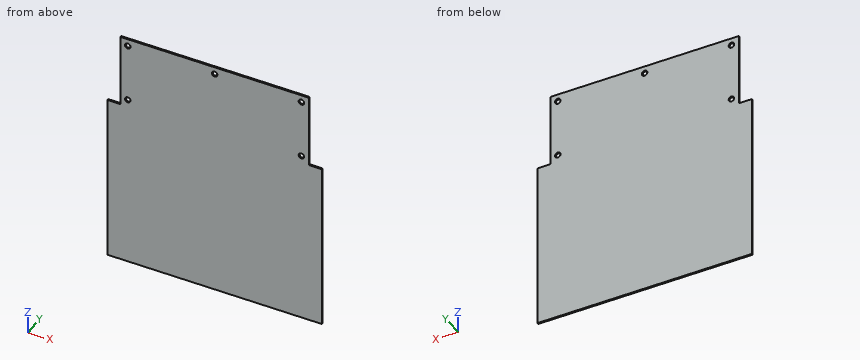
from build123d import *

# Parameters (mm, degrees)
F0_R     = 3.25
F1_DEPTH = 2
F2_SIZE  = 0.5


with BuildPart() as f1:
    # F0 (on Front) → F1 (new body)
    with BuildSketch(Plane.XZ):
        Polygon((145, -115), (145, 115), (127.5, 115), (127.5, 215), (-127.5, 215), (-127.5, 115), (-145, 115), (-145, -115), align=None)
        with Locations((-117.5, 125)):
            Circle(F0_R, mode=Mode.SUBTRACT)
        with Locations((-117.5, 205)):
            Circle(F0_R, mode=Mode.SUBTRACT)
        with Locations((117.5, 125)):
            Circle(F0_R, mode=Mode.SUBTRACT)
        with Locations((0, 205)):
            Circle(F0_R, mode=Mode.SUBTRACT)
        with Locations((117.5, 205)):
            Circle(F0_R, mode=Mode.SUBTRACT)
    extrude(amount=F1_DEPTH)

    # F2
    f2_edges = [f1.edges().sort_by_distance(p)[0] for p in [
        (-114.25, -1, 125),
        (-120.75, 0, 125),
        (-120.75, -2, 125),
        (-114.25, -1, 205),
        (-120.75, 0, 205),
        (-120.75, -2, 205),
        (120.75, -1, 205),
        (114.25, 0, 205),
        (114.25, -2, 205),
        (120.75, -1, 125),
        (114.25, 0, 125),
        (114.25, -2, 125),
        (3.25, -1, 205),
        (-3.25, 0, 205),
        (-3.25, -2, 205),
    ]]
    chamfer(f2_edges, length=F2_SIZE)


solid = f1.part
Can you work these out from the model? Positions are in its coordinate system, mm. Give positions to 0.01 mm unless a question says otherwise; leave off trailing zeros. Order: outer loops, then holes, each group sorted by start corner. A loop starts at its lowest first (then second) coordinate and runs counter-clockwise, first axis right, second up. Notation, with made-up numbers: M -11.75,-28.75 L 38.25,-28.75 A23 cw 38.25,-4.75 Z; hole C 15,-3.75 d8. An arc over 180 degrees is marked long. Use one line per item in the form item = value. Start each with the question number.
Item 1: If we section it at A-A (y = -0.8): Write out the boundary of the cut face in (x, z).
Item 2: If I drill on line 1 along Z through (x, y) = (-117.5, -0.9); line 2 along X through (y, z) = (-1.1, 205); line 3 along X through (y, z) = (-0.85, 199.5), over which ranges is the centre line in solid material (lowest first)?
Item 3: If we section it at B-B (z = 145): Write out the boundary of the cut face in (x, y).
Item 4: Will this pin go through, and if not, where does the flat tip stop? pin 1 Ø0.6 at (y, z) = (-1, 175.5) entering from -X.
Outcome:
q1.outline = M -145,-115 L 145,-115 L 145,115 L 127.5,115 L 127.5,215 L -127.5,215 L -127.5,115 L -145,115 Z; hole C -117.5,125 d6.5; hole C -117.5,205 d6.5; hole C 0,205 d6.5; hole C 117.5,125 d6.5; hole C 117.5,205 d6.5
q2.line_1 = -115 to 121.75, 128.25 to 201.75, 208.25 to 215
q2.line_2 = -127.5 to -120.75, -114.25 to -3.25, 3.25 to 114.25, 120.75 to 127.5
q2.line_3 = -127.5 to 127.5
q3.outline = M -127.5,-2 L 127.5,-2 L 127.5,0 L -127.5,0 Z
q4.pin_1 = -127.5
